The listing builds one solid part. Answer for the finished solid, in the listing's coordinates (mm). A direction names the side the tool comes from. Round coordinates to 2 decimals unless told otherwise and drop trailing zeros. Order: outer loops, then holes, each group sorted by start corner. A loop starts at its lowest first (then second) coordinate and runs counter-clockwise, first axis right, second up. Notation, with made-up numbers: (84.25, 58.25) -> (108.25, 58.25) arc R30 ccw to (108.25, 94.25) -> close; hole circle Ø11 at (-27.5, -36). An arc over 180 degrees is marked (long way). Return JSON: item names as keys, results as strings. Group by question number.
(1) Each of these flat-tipped pins is pushed along its axis until it touches: pin 1 (5 mm diameter, centred on x = 90.5, y = 19.5, fed in from -Z); pin 2 (8.5 mm diameter, centred on x = 51.5, z = 67.5, fed in from -Y); pin 3 (0.5 mm diameter, centred on y = 33.5, z = -44.5, fed in from -X); pin 4 (6 mm diameter, centred on x = 136.5, y = 8.5, fed in from -Z). Where does it stop, or does it pass through?
(2) Consider line 1 (Y direction, x = 141, z = 27); line 2 (Z direction, x = 13, y = 43); line 3 (Z direction, x = 186, y = 14) (3 decimals). Determine where each line is inside the solid, lowest interval first. Write a range as [from, to].
(3) Determine the mould class of faces 1 (the face through (229.064, 41.821, 23.706)), 2 (the face through (150.699, 50.076, -59.931)) for opening direction Z: +Z half, -Z half, draft (parallel to the pull), parting line (faces both ways), or undercut.
(4) The part is cut by section A-A (y = 39). Determine the outline of the cut face in (x, z) (3 decimals).
(5) Which of the six approach directions +Z, -Z, +X, -X, +Y, -Y give full straight-line access (tool end or side, diameter ignored) to faces 3 (the face through (155.065, 25.08, -59.714)), 4 (the face through (229.469, 13.424, -22.83)), 5 (the face through (62.31, 32.43, 61.66))?
from build123d import *

# Parameters (mm, degrees)
BOSS_EXTRUDE1_DEPTH = 12.7
BOSS_EXTRUDE2_DEPTH = 38.1
SKETCH3_W           = 48.711101319
SKETCH3_H           = 95.25
CUT_EXTRUDE1_DEPTH  = 38.1
FILLET1_R           = 2.54
BOSS_EXTRUDE3_DEPTH = 6.35


with BuildPart() as part:
    # Sketch1 → Boss-Extrude1 (new body)
    with BuildSketch(Plane(origin=(0, 0, 0), x_dir=(1, 0, 0), z_dir=(0, 1, 0))):
        Polygon((0, 95.25), (0, -95.25), (304.8, -25.4), (304.8, 25.4), align=None)
    extrude(amount=BOSS_EXTRUDE1_DEPTH)

    # Sketch2 → Boss-Extrude2 (add)
    with BuildSketch(Plane(origin=(0, 12.7, 0), x_dir=(1, 0, 0), z_dir=(0, 1, 0))):
        Polygon((0, 76.2), (304.8, 6.35), (304.8, 25.4), (0, 95.25), align=None)
        Polygon((304.8, -6.35), (0, -76.2), (0, -95.25), (304.8, -25.4), align=None)
    extrude(amount=BOSS_EXTRUDE2_DEPTH)

    # Sketch3 → Cut-Extrude1 (cut)
    with BuildSketch(Plane(origin=(0, 50.8, 0), x_dir=(1, 0, 0), z_dir=(0, 1, 0))):
        with Locations((128.044449341, 0)):
            Rectangle(SKETCH3_W, SKETCH3_H)
    extrude(amount=-CUT_EXTRUDE1_DEPTH, mode=Mode.SUBTRACT)

    # Fillet1
    fillet1_edges = [part.edges().sort_by_distance(p)[0] for p in [
        (304.8, 12.7, 0),
        (228.6, 12.7, 23.8125),
        (304.8, 31.75, 6.35),
        (0, 31.75, 76.2),
        (304.8, 50.8, 15.875),
        (228.6, 50.8, 23.8125),
        (0, 50.8, 85.725),
        (152.4, 50.8, 60.325),
        (0, 12.7, 0),
        (62.345454545, 12.7, -61.9125),
        (0, 31.75, -76.2),
        (304.8, 31.75, -6.35),
        (0, 50.8, -85.725),
        (62.345454545, 50.8, -61.9125),
        (304.8, 50.8, -15.875),
        (152.4, 50.8, -60.325),
        (228.6, 50.8, -23.8125),
        (152.4, 50.8, -44.45),
        (228.6, 12.7, -23.8125),
        (62.345454545, 50.8, 61.9125),
        (62.345454545, 12.7, 61.9125),
        (124.690909091, 31.75, 47.625),
        (152.4, 31.75, 47.625),
        (138.545454545, 50.8, 47.625),
        (152.4, 50.8, 44.45),
        (138.545454545, 50.8, -47.625),
        (152.4, 12.7, 44.45),
        (138.545454545, 12.7, 47.625),
        (138.545454545, 12.7, -47.625),
        (152.4, 12.7, -44.45),
        (152.4, 31.75, 41.275),
        (152.4, 31.75, -41.275),
        (152.4, 31.75, -47.625),
        (124.690909091, 31.75, -47.625),
        (304.8, 0, 0),
        (152.4, 0, 60.325),
        (0, 0, 0),
        (152.4, 0, -60.325),
        (304.8, 25.4, -25.4),
        (304.8, 25.4, 25.4),
        (0, 25.4, 95.25),
        (0, 25.4, -95.25),
    ]]
    fillet(fillet1_edges, radius=FILLET1_R)

    # Sketch4 → Boss-Extrude3 (add)
    with BuildSketch(Plane(origin=(0, 35.56, 0), x_dir=(1, 0, 0), z_dir=(0, 1, 0))):
        Polygon((301.692624563, -7.062106871), (154.372624563, -40.822940204), (154.372624563, -40.562355842), (301.635887019, -6.814524862), align=None)
        Polygon((124.410851298, -47.689179911), (1.972624563, -75.747940204), (1.972624563, -75.487355842), (124.354113754, -47.441597902), align=None)
        Polygon((154.372624563, 40.822940204), (301.692624563, 7.062106871), (301.635887019, 6.814524862), (154.315887019, 40.575358195), align=None)
        Polygon((1.972624563, 75.747940204), (124.410851298, 47.689179911), (124.354113754, 47.441597902), (1.915887019, 75.500358195), align=None)
    extrude(amount=-BOSS_EXTRUDE3_DEPTH)


solid = part.part
Answer below:
{
 "1": {"pin 1": "stops at z = -75.08", "pin 2": "stops at y = 0", "pin 3": "stops at x = 152.4", "pin 4": "stops at z = -64.66"},
 "2": {"line 1": "y = [0, 12.7]", "line 2": "z = [-92.27, -73.22], [73.22, 92.27]", "line 3": "z = [-52.625, -33.243], [33.243, 52.625]"},
 "3": {"face 1": "undercut", "face 2": "-Z half"},
 "4": {"outline": "(0, -92.062) arc R2.54 ccw to (3.107, -94.538) -> (302.827, -25.852) arc R2.54 ccw to (304.8, -23.376) -> (304.8, -9.538) arc R2.54 ccw to (301.693, -7.062) -> (154.373, -40.823) arc R2.54 ccw to (152.4, -43.299) -> (152.4, -45.085) arc R2.54 cw to (149.86, -47.625) -> (124.978, -47.625) arc R2.54 ccw to (124.411, -47.689) -> (1.973, -75.748) arc R2.54 ccw to (0, -78.224) -> close; (0, 78.224) arc R2.54 ccw to (1.973, 75.748) -> (124.411, 47.689) arc R2.54 ccw to (124.978, 47.625) -> (149.86, 47.625) arc R2.54 cw to (152.4, 45.085) -> (152.4, 43.299) arc R2.54 ccw to (154.373, 40.823) -> (301.693, 7.062) arc R2.54 ccw to (304.8, 9.538) -> (304.8, 23.376) arc R2.54 ccw to (302.827, 25.852) -> (3.107, 94.538) arc R2.54 ccw to (0, 92.062) -> close"},
 "5": {"face 3": "-Z, +X, +Y, -Y", "face 4": "-X", "face 5": "-X, +Y"}
}
